```python
from build123d import *

# Parameters (mm, degrees)
PROFILEEXTRUDE_DEPTH    = 73.76
HOSEWINDOW_W            = 16.29
HOSEWINDOW_H            = 26.5
HOSEWINDOWCUT_DEPTH     = 23.11
CAGESCREWS_R            = 2.4
CAGESCREWSCUT_DEPTH     = 23.11
AXLEHOLECUT_DEPTH       = 23.11
SETSCREWHOLES_R         = 1.539432213
SETSCREWHOLES_R_2       = 1.628953018
SETSCREWHOLESCUT_DEPTH  = 23.11
VELOCITYWINDOW_W        = 12.61
VELOCITYWINDOW_H        = 22.29
VELOCITYWINDOWCUT_DEPTH = 23.11
FILLET3_R               = 7
TRIGGERRACKSLOTCUT_W    = 6.35
TRIGGERRACKSLOTCUT_H    = 6.35
RACKSLOTCUT_DEPTH       = 23.11
FILLET4_R               = 1


with BuildPart() as part:
    # Profile → ProfileExtrude (new body)
    with BuildSketch(Plane.XY):
        with BuildLine():
            Line((9.301269376, -54.194713793), (9.301269376, -29.194713793))
            Line((9.301269376, -29.194713793), (-0.848730624, -29.194713793))
            Line((-0.848730624, -29.194713793), (-0.848730624, -13.196583793))
            ThreePointArc((-0.848730624, -13.196583793), (-4.204324299, -9.619560571), (-6.340730624, -5.204713793))
            Line((-6.340730624, -5.204713793), (-8.928730624, -5.204713793))
            Line((-8.928730624, -5.204713793), (-8.928730624, 6.495286207))
            Line((-8.928730624, 6.495286207), (-6.509650624, 6.495286207))
            ThreePointArc((-6.509650624, 6.495286207), (-4.210311879, 9.168674207), (-1.388730624, 11.283536207))
            Line((-1.388730624, 11.283536207), (-1.388730624, 21.845286207))
            Line((-1.388730624, 21.845286207), (10.261269376, 21.845286207))
            Line((10.261269376, 21.845286207), (10.261269376, 31.845286207))
            Line((10.261269376, 31.845286207), (-11.848730624, 31.845286207))
            Line((-11.848730624, 31.845286207), (-11.848730624, -54.194713793))
            Line((-11.848730624, -54.194713793), (9.301269376, -54.194713793))
        make_face()
    extrude(amount=PROFILEEXTRUDE_DEPTH)

    # HoseWindow → HoseWindowCut (cut, through all)
    with BuildSketch(Plane.ZY.offset(11.848730624)):
        with Locations((56.725, -40.944713793)):
            Rectangle(HOSEWINDOW_W, HOSEWINDOW_H)
    extrude(amount=-HOSEWINDOWCUT_DEPTH, mode=Mode.SUBTRACT)

    # CageScrews → CageScrewsCut (cut, through all)
    with BuildSketch(Plane.ZY.offset(11.848730624)):
        with Locations((7.5, 26.845286207)):
            Circle(CAGESCREWS_R)
        with Locations((66.26, 26.845286207)):
            Circle(CAGESCREWS_R)
        with Locations((7.5, -49.194713793)):
            Circle(CAGESCREWS_R)
        with Locations((69.31, -49.194713793)):
            Circle(CAGESCREWS_R)
    extrude(amount=-CAGESCREWSCUT_DEPTH, mode=Mode.SUBTRACT)

    # AxleHole → AxleHoleCut (cut, through all)
    with BuildSketch(Plane.ZY.offset(11.848730624)):
        with BuildLine():
            Line((47.361, 8.359497151), (47.361, 6.740497151))
            Line((47.361, 6.740497151), (44.699, 6.740497151))
            Line((44.699, 6.740497151), (44.699, 8.359497151))
            ThreePointArc((44.699, 8.359497151), (46.03, -4.783713793), (47.361, 8.359497151))
        make_face()
    extrude(amount=-AXLEHOLECUT_DEPTH, mode=Mode.SUBTRACT)

    # SetScrewHoles → SetScrewHolesCut (cut, through all)
    with BuildSketch(Plane.ZY.offset(11.848730624)):
        with Locations((6.03, 1.855286207)):
            Circle(SETSCREWHOLES_R)
        with Locations((68.03, 1.855286207)):
            Circle(SETSCREWHOLES_R_2)
    extrude(amount=-SETSCREWHOLESCUT_DEPTH, mode=Mode.SUBTRACT)

    # VelocityWindow → VelocityWindowCut (cut, through all)
    with BuildSketch(Plane.ZY.offset(11.848730624)):
        with Locations((32.655, -15.499713793)):
            Rectangle(VELOCITYWINDOW_W, VELOCITYWINDOW_H)
    extrude(amount=-VELOCITYWINDOWCUT_DEPTH, mode=Mode.SUBTRACT)

    # Fillet3
    fillet3_edges = [part.edges().sort_by_distance(p)[0] for p in [
        (-11.848730624, -26.644713793, 32.655),
    ]]
    fillet(fillet3_edges, radius=FILLET3_R)

    # TriggerRackSlotCut → RackSlotCut (cut, through all)
    with BuildSketch(Plane.ZY.offset(11.848730624)):
        with Locations((18.175, -44.669713793)):
            Rectangle(TRIGGERRACKSLOTCUT_W, TRIGGERRACKSLOTCUT_H)
        with Locations((30.875, -44.669713793)):
            Rectangle(TRIGGERRACKSLOTCUT_W, TRIGGERRACKSLOTCUT_H)
        with Locations((5.475, -31.969713793)):
            Rectangle(TRIGGERRACKSLOTCUT_W, TRIGGERRACKSLOTCUT_H)
        with Locations((18.175, -31.969713793)):
            Rectangle(TRIGGERRACKSLOTCUT_W, TRIGGERRACKSLOTCUT_H)
        with Locations((5.475, -16.969713793)):
            Rectangle(TRIGGERRACKSLOTCUT_W, TRIGGERRACKSLOTCUT_H)
        with Locations((18.175, -16.969713793)):
            Rectangle(TRIGGERRACKSLOTCUT_W, TRIGGERRACKSLOTCUT_H)
    extrude(amount=-RACKSLOTCUT_DEPTH, mode=Mode.SUBTRACT)

    # Fillet4
    fillet4_edges = [part.edges().sort_by_distance(p)[0] for p in [
        (-11.848730624, -11.174713793, 73.76),
        (-11.848730624, -18.999713793, 26.35),
        (-11.848730624, -18.999713793, 38.96),
        (-11.848730624, -4.354713793, 32.655),
        (-11.848730624, -44.669713793, 15),
        (-11.848730624, -47.844713793, 18.175),
        (-11.848730624, -44.669713793, 21.35),
        (-11.848730624, -41.494713793, 18.175),
        (-11.848730624, -11.174713793, 0),
        (-11.848730624, -31.969713793, 2.3),
        (-11.848730624, -35.144713793, 5.475),
        (-11.848730624, -31.969713793, 8.65),
        (-11.848730624, -28.794713793, 5.475),
        (-11.848730624, -44.669713793, 27.7),
        (-11.848730624, -47.844713793, 30.875),
        (-11.848730624, -44.669713793, 34.05),
        (-11.848730624, -41.494713793, 30.875),
        (-11.848730624, -31.969713793, 15),
        (-11.848730624, -35.144713793, 18.175),
        (-11.848730624, -31.969713793, 21.35),
        (-11.848730624, -28.794713793, 18.175),
        (-11.848730624, -54.194713793, 69.315),
        (-11.848730624, 31.845286207, 36.88),
        (-11.848730624, -16.969713793, 2.3),
        (-11.848730624, -20.144713793, 5.475),
        (-11.848730624, -16.969713793, 8.65),
        (-11.848730624, -13.794713793, 5.475),
        (-11.848730624, -16.969713793, 15),
        (-11.848730624, -20.144713793, 18.175),
        (-11.848730624, -16.969713793, 21.35),
        (-11.848730624, -13.794713793, 18.175),
        (-11.848730624, -54.194713793, 24.29),
        (-11.848730624, -40.944713793, 64.87),
        (-11.848730624, -27.694713793, 56.725),
        (-11.848730624, -40.944713793, 48.58),
    ]]
    fillet(fillet4_edges, radius=FILLET4_R)


solid = part.part
```
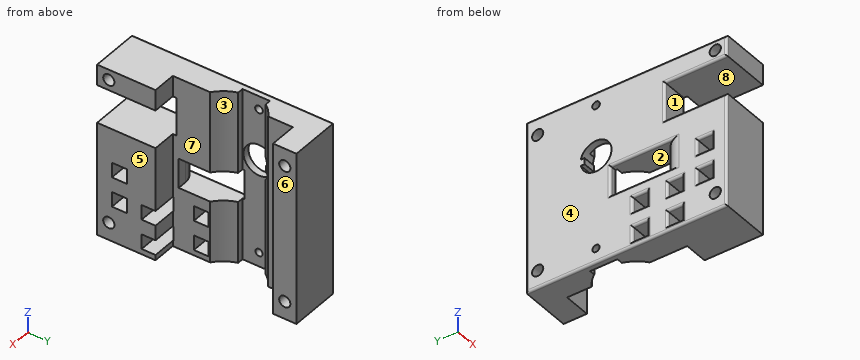
Design review of the part built by this model. Coordinates are the model's own, in mm. Face numbers are marked on the shaded views. A direction names the side the tool comes from. Coordinates: 2 decimals unless noted, no trailing zeros. Loops run counter-clockwise (first coordinate to the right, second up) from the corner with the lowest first, then second, coordinate; pieces in that order, holes last.
Q1. To check wall thickness, follow line 1 (Z direction, x = -8, y = -31.5); line 2 (Z direction, x = -4.25, y = -19); line 3 (Z direction, x = -7.5, y = -35.5). State the ranges of each line that lie inside material, in increasing order.
Reported:
line 1: z = 0 to 2.3, 8.65 to 15, 21.35 to 48.58, 64.87 to 73.76
line 2: z = 0 to 2.3, 8.65 to 15, 21.35 to 26.35, 38.96 to 73.76
line 3: z = 0 to 48.58, 64.87 to 73.76
Q2. We need section A-A on y = -16.5. State the section outline as (x, z) points.
Reported:
outline: (-11.85, 1) arc R1 ccw to (-10.85, 0) - (-0.85, 0) - (-0.85, 2.3) - (-10.85, 2.3) arc R1 ccw to (-11.85, 1.3) - close; (-11.85, 9.65) arc R1 ccw to (-10.85, 8.65) - (-0.85, 8.65) - (-0.85, 15) - (-10.85, 15) arc R1 ccw to (-11.85, 14) - close; (-11.85, 22.35) arc R1 ccw to (-10.85, 21.35) - (-0.85, 21.35) - (-0.85, 26.35) - (-10.85, 26.35) arc R1 ccw to (-11.85, 25.35) - close; (-11.85, 39.96) arc R1 ccw to (-10.85, 38.96) - (-0.85, 38.96) - (-0.85, 73.76) - (-10.85, 73.76) arc R1 ccw to (-11.85, 72.76) - close
Q3. Tool access review of the marked faces 5, 6, 7 and 8: name each direction out of +Z, -Z, +X, -X, +Y, -Y from which nothing blocks a thin tool from reaching the whole face with its end or side.
Reported:
face 5: +Z, -Z, +X, -Y
face 6: +Z, -Z, +X, +Y, -Y
face 7: +Z, -Z, +X
face 8: +X, -X, -Y
Q4. For pin 1 (3 mm diameter, centred on y = -4.5, z = 22, fed in from +X); pin 2 (3.5 mm diameter, centred on y = 1.86, z = 6.03, fed in from +X); pin 3 (3 mm diameter, centred on x = 5.5, z = 52.5, fed in from -Y), all flat-tipped, find the tip position at first contact; note any pin that passes through.
Reported:
pin 1: stops at x = -6.07
pin 2: stops at x = -8.93
pin 3: stops at y = 21.85
Q5. The part is to be moulded in two halves that separate along Y. For the marked faces 1, 2, 3 and 4, say which applies: +Y half, -Y half, draft (parallel to the pull), parting line (faces both ways), or undercut.
Reported:
face 1: -Y half
face 2: undercut
face 3: undercut
face 4: draft
Q6. We need section B-B on z = 16. State how many separate pieces and enclosed holes the cut face has, and give its area (3 significant figures).
Reported:
separate pieces: 4
enclosed holes: 0
area: 832 mm2
Q7. We need section D-D on z = 46.03. State the section outline as (x, y) points.
Reported:
outline: (-11.85, -53.19) arc R1 ccw to (-10.85, -54.19) - (9.3, -54.19) - (9.3, -29.19) - (-0.85, -29.19) - (-0.85, -13.2) arc R16.26 cw to (-6.34, -5.2) - (-8.93, -5.2) - (-8.93, -4.78) - (-11.85, -4.78) - close; (-11.85, 6.74) - (-6.34, 6.74) arc R16.26 cw to (-1.39, 11.28) - (-1.39, 21.85) - (10.26, 21.85) - (10.26, 31.85) - (-10.85, 31.85) arc R1 ccw to (-11.85, 30.85) - close
